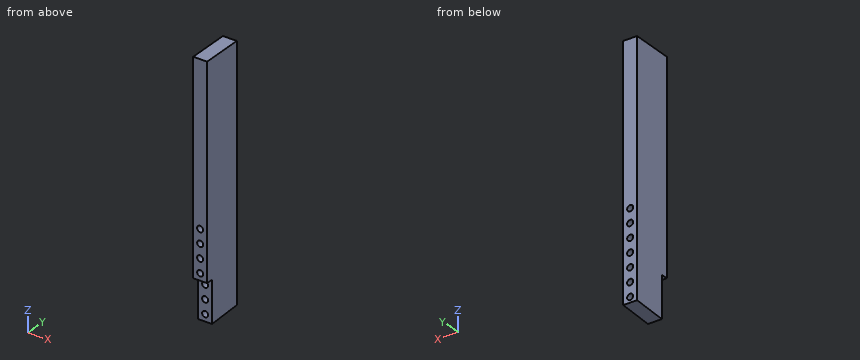
```python
from build123d import *

# Parameters (mm, degrees)
F1_DEPTH = 12.7
F2_R     = 5.55625
F3_DEPTH = 63.501
F4_R     = 5.55625
F5_DEPTH = 76.201


with BuildPart() as f1:
    # F0 (on Right) → F1 (new body, symmetric)
    with BuildSketch(Plane.YZ):
        Polygon((76.2, 457.2), (0, 457.2), (0, 76.2), (12.7, 76.2), (12.7, 0), (76.2, 2.77247), align=None)
    extrude(amount=F1_DEPTH, both=True)

    # F2 (on face) → F3 (cut, through all)
    with BuildSketch(Plane.XZ.offset(-12.7)):
        with Locations((0, 38.1)):
            Circle(F2_R)
        with Locations((0, 63.5)):
            Circle(F2_R)
        with Locations((0, 12.7)):
            Circle(F2_R)
    extrude(amount=-F3_DEPTH, mode=Mode.SUBTRACT)

    # F4 (on face) → F5 (cut, through all)
    with BuildSketch(Plane.XZ):
        with Locations((0, 114.3)):
            Circle(F4_R)
        with Locations((0, 139.7)):
            Circle(F4_R)
        with Locations((0, 88.9)):
            Circle(F4_R)
        with Locations((0, 165.1)):
            Circle(F4_R)
    extrude(amount=-F5_DEPTH, mode=Mode.SUBTRACT)


solid = f1.part
```
Input: part model. Units: mm. Frame: model coordinates. Coordinates: 2 decimals unless noted, no trailing zeros. Order: outer loops, then holes, each group sorted by start corner. A loop starts at its lowest first (then second) coordinate and runs counter-clockwise, first axis right, second up. Notation, with made-up numbers: (-12.5, -6) - (22.5, -6) arc R15 ccw to (22.5, 2) - close; hole circle Ø11 at (45.5, -8.75). An arc over 180 degrees is marked (long way). Put each result on its own line as item: value.
1. Contact query for flat-ended pins moving along their axis: pin 1 Ø9 at (x, z) = (0, 38.1) entering from +Y; pin 2 Ø4 at (x, y) = (5, 53.5) entering from -Z; pin 3 Ø12.5 at (x, z) = (1, 24.5) entering from -Y; pin 4 Ø10 at (x, y) = (-5.5, 5.5) entering from -Z. Output: stop coordinate, or through.
Report:
pin 1: passes through
pin 2: stops at z = 1.69
pin 3: stops at y = 12.7
pin 4: stops at z = 76.2
2. Cut plane B-B on x = 0. State how many separate pieces and enclosed holes the cut face has, then the cut area to 3 significant figures.
Report:
separate pieces: 8
enclosed holes: 0
area: 28,300 mm2
3. Cut plane C-C on z = 88.9. Return the cut outline in (x, y).
Report:
outline: (-12.7, 0) - (-5.56, 0) - (-5.56, 76.2) - (-12.7, 76.2) - close; (5.56, 0) - (12.7, 0) - (12.7, 76.2) - (5.56, 76.2) - close
4. Line query: line 1 along Z through (x, y) = (3.75, 11.5); line 2 along X through (y, z) = (46, 63); line 3 along Y through (x, z) = (-6.25, 27.5). Output: solid intervals per line, ascending.
Report:
line 1: z = 76.2 to 84.8, 93 to 110.2, 118.4 to 135.6, 143.8 to 161, 169.2 to 457.2
line 2: x = -12.7 to -5.53, 5.53 to 12.7
line 3: y = 12.7 to 76.2
5. Cut plane A-A on z = 38.1. Return the cut outline in (x, y).
Report:
outline: (-12.7, 12.7) - (-5.56, 12.7) - (-5.56, 76.2) - (-12.7, 76.2) - close; (5.56, 12.7) - (12.7, 12.7) - (12.7, 76.2) - (5.56, 76.2) - close
